```python
from build123d import *

# Parameters (mm, degrees)
SKETCH1_W           = 108
SKETCH1_H           = 164
BOSS_EXTRUDE1_DEPTH = 2
SKETCH2_R           = 22
CUT_EXTRUDE1_DEPTH  = 1
SKETCH3_R           = 20
CUT_EXTRUDE2_DEPTH  = 2


with BuildPart() as part:
    # Sketch1 → Boss-Extrude1 (new body)
    with BuildSketch(Plane(origin=(0, 0, 0), x_dir=(1, 0, 0), z_dir=(0, 1, 0))):
        Rectangle(SKETCH1_W, SKETCH1_H)
    extrude(amount=-BOSS_EXTRUDE1_DEPTH)

    # Sketch2 → Cut-Extrude1 (cut)
    with BuildSketch(Plane(origin=(0, 0, 0), x_dir=(1, 0, 0), z_dir=(0, 1, 0))):
        Circle(SKETCH2_R)
    extrude(amount=-CUT_EXTRUDE1_DEPTH, mode=Mode.SUBTRACT)

    # Sketch3 → Cut-Extrude2 (cut, through all)
    with BuildSketch(Plane(origin=(0, -1, 0), x_dir=(1, 0, 0), z_dir=(0, 1, 0))):
        Circle(SKETCH3_R)
    extrude(amount=-CUT_EXTRUDE2_DEPTH, mode=Mode.SUBTRACT)


solid = part.part
```
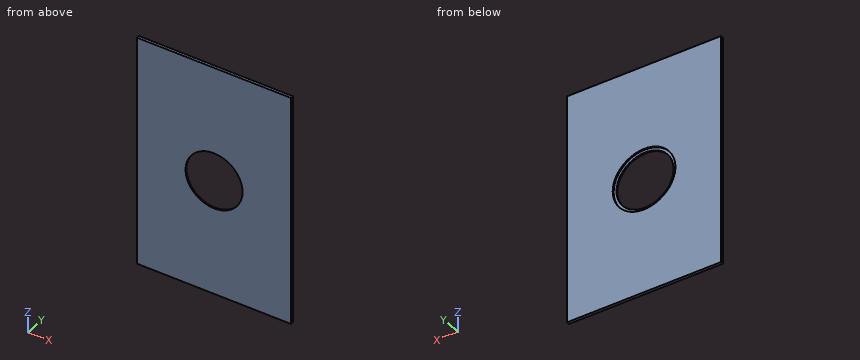
Geometry check sheet. Reference: the model listing, model coordinates, mm. Coordinates: 2 decimals unless noted, no trailing zeros. Write each loop counter-clockwise with the first axis right and the second up, starting at its lowest first coordinate (ties: lowest second). Pieces come first, ordered by that corner, then holes. Notation, with made-up numbers: (-27, 22) -> (22, 22) arc R17 cw to (22, 52) -> close; hole circle Ø10 at (65.25, 75.25). An arc over 180 degrees is marked (long way). Use CSV: the item, a comma, the result in double quotes. Start each with the question number.
Item 1: Cross-section at C-C, the plane y = -0.4. Record the cut outline in (x, z), plus the area to 3 significant figures.
Item 2: Depth check by flat-ended pin: pin 1 Ø1.5 at (x, z) = (0.5, 18) entering from +Y. Enter the tip coordinate at first touch or a pass-through.
Item 3: Cross-section at A-A, the plane x = 0. Record the cut outline in (y, z), plus the area to 3 significant figures.
Item 4: Thickness scan on line 1 (X direction, y = -0.8, z = 0); line 2 (Z direction, x = 0, y = -1.65); line 3 (X direction, y = -1.25, z = 0). Record the ranges inside material, lowest first.
Item 5: Cross-section at B-B, the plane z = 0. Record the cut outline in (x, y), plus the area to 3 significant figures.
Answers:
1,outline,"(-54, -82) -> (54, -82) -> (54, 82) -> (-54, 82) -> close; hole circle Ø44 at (0, 0)"
1,area,"16,200 mm^2"
2,pin 1,"through"
3,outline,"(-2, -82) -> (0, -82) -> (0, -22) -> (-1, -22) -> (-1, -20) -> (-2, -20) -> close; (-2, 20) -> (-1, 20) -> (-1, 22) -> (0, 22) -> (0, 82) -> (-2, 82) -> close"
3,area,"244 mm^2"
4,line 1,"-54 to -22, 22 to 54"
4,line 2,"-82 to -20, 20 to 82"
4,line 3,"-54 to -20, 20 to 54"
5,outline,"(-54, -2) -> (-20, -2) -> (-20, -1) -> (-22, -1) -> (-22, 0) -> (-54, 0) -> close; (20, -2) -> (54, -2) -> (54, 0) -> (22, 0) -> (22, -1) -> (20, -1) -> close"
5,area,"132 mm^2"
